from build123d import *

# Parameters (mm, degrees)
ESQUISSE1_W      = 7
ESQUISSE1_H      = 2
EXTRUSION1_DEPTH = 7
ESQUISSE2_R      = 0.25
EXTRUSION2_DEPTH = 3


with BuildPart() as part:
    # Esquisse1 → Extrusion1 (new body)
    with BuildSketch(Plane(origin=(0, 0, 0), x_dir=(1, 0, 0), z_dir=(0, 1, 0))):
        with Locations((3.5, 1)):
            Rectangle(ESQUISSE1_W, ESQUISSE1_H)
    extrude(amount=EXTRUSION1_DEPTH)

    # Esquisse2 → Extrusion2 (add)
    with BuildSketch(Plane.XZ):
        with Locations(Location((0.96, -1, 0), (0, 0, 90))):
            Circle(ESQUISSE2_R)
        with Locations(Location((6.04, -1, 0), (0, 0, 270))):
            Circle(ESQUISSE2_R)
    extrude(amount=EXTRUSION2_DEPTH)


solid = part.part
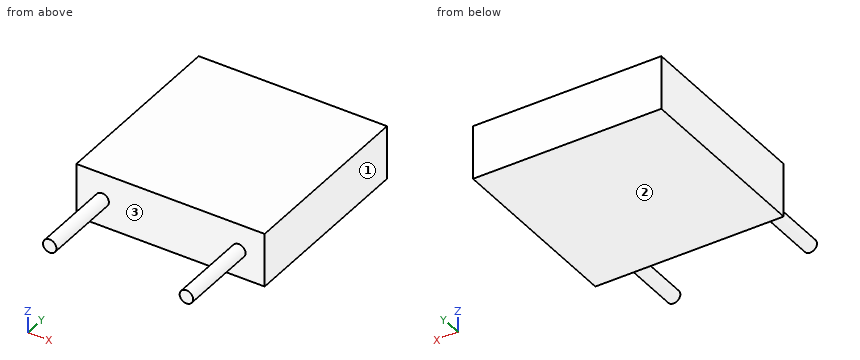
CAD build for the part. Positions are in the model's coordinates, mm. Face numbers are marked on the shaded views. Give positions to 0.01 mm unless a question says otherwise; leave off trailing zeros. Write each loop counter-clockwise with the first axis right and the second up, starting at its lowest first coordinate (ties: lowest second). Pieces come first, ordered by that corner, then holes. Notation, with made-up numbers: (30, 72.5) - (37, 72.5) arc R16 cw to (37, 98.5) - close; hole circle Ø2 at (-27.75, 71.5). An arc over 180 degrees is marked (long way). Put each result on its own line as item: value.
(1) Saw through at D-D (z = -0.1). List the corners of the cut face in (x, y), then the cut area to 3 significant figures.
Working result:
outline: (0, 0) - (7, 0) - (7, 7) - (0, 7) - close
area: 49.0 mm^2
(2) Saw through at B-B (z = -1). List the corners of the cut face in (x, y).
Working result:
outline: (0, 0) - (0.71, 0) - (0.71, -3) - (1.21, -3) - (1.21, 0) - (5.79, 0) - (5.79, -3) - (6.29, -3) - (6.29, 0) - (7, 0) - (7, 7) - (0, 7) - close
(3) Saw through at A-A (x = 0.96). List the corners of the cut face in (y, z).
Working result:
outline: (-3, -1.25) - (0, -1.25) - (0, -2) - (7, -2) - (7, 0) - (0, 0) - (0, -0.75) - (-3, -0.75) - close
(4) Saw through at C-C (x = 4.5). List the corners of the cut face in (y, z).
Working result:
outline: (0, -2) - (7, -2) - (7, 0) - (0, 0) - close
(5) Wall check: L1, parallel to Y at x = 5, z = -0.75; L2, parallel to Z at x = 6, y = -1; L3, parallel to X at y = -1.25, z = -0.85. Give the ranges that are in metal, low to high.
Working result:
L1: 0 to 7
L2: -1.25 to -0.75
L3: 0.76 to 1.16, 5.84 to 6.24
(6) Pull direction X, two halves, no side cores. Call the marked faces 1, 2 and 3: released by +X, released by -X, zero draft, split by the parting line, or undercut.
Working result:
face 1: released by +X
face 2: zero draft
face 3: undercut
